Can you work these out from the model? Positions are in its coordinate system, mm. A direction names the side the tool comes from. Coordinates: 2 decimals unless noted, no trailing zeros. Write each loop counter-clockwise with the first axis right and the second up, starting at its lowest first coordinate (ties: lowest second). Pieces come first, ordered by that corner, then holes. Notation, with made-up numbers: M -13.75,26.25 L 16.25,26.25 A24 cw 16.25,40.25 Z; hole C 65.25,8.5 d6. An arc over 180 degrees is marked long. Answer as a JSON object with one key per item and string values. Group by question number.
from build123d import *

# Parameters (mm, degrees)
EXTRUDE_1_DEPTH     = 1.5
SKETCH_2_R          = 0.85
CUT_EXTRUDE_1_DEPTH = 11
SKETCH_4_R          = 0.85
CUT_EXTRUDE_2_DEPTH = 11.5
SKETCH_5_R          = 0.85
CUT_EXTRUDE_3_DEPTH = 11.5
SKETCH_9_R          = 1.55
SKETCH_9_R_2        = 0.85
CUT_EXTRUDE_5_DEPTH = 1
SKETCH_8_R          = 1.75
SKETCH_8_R_2        = 0.85
EXTRUDE_6_DEPTH     = 8.6
FILLET_2_R          = 1


with BuildPart() as part:
    # 草图1 → 凸台-拉伸1 (new body)
    with BuildSketch(Plane.XY):
        with BuildLine():
            Line((-26.273021583, 44.286870504), (15.826978417, 44.286870504))
            ThreePointArc((15.826978417, 44.286870504), (22.332360804, 41.592252891), (25.026978417, 35.086870504))
            Line((25.026978417, 35.086870504), (25.026978417, -7.013129496))
            ThreePointArc((25.026978417, -7.013129496), (22.332360804, -13.518511883), (15.826978417, -16.213129496))
            Line((15.826978417, -16.213129496), (-26.273021583, -16.213129496))
            ThreePointArc((-26.273021583, -16.213129496), (-32.77840397, -13.518511883), (-35.473021583, -7.013129496))
            Line((-35.473021583, -7.013129496), (-35.473021583, 35.086870504))
            ThreePointArc((-35.473021583, 35.086870504), (-32.77840397, 41.592252891), (-26.273021583, 44.286870504))
        make_face()
    extrude(amount=EXTRUDE_1_DEPTH)

    # 草图2 → 切除-拉伸1 (cut)
    with BuildSketch(Plane.XY.offset(1.5)):
        with Locations((-27.773021583, 36.586870504)):
            Circle(SKETCH_2_R)
    extrude(amount=-CUT_EXTRUDE_1_DEPTH, mode=Mode.SUBTRACT)

    # 草图4 → 切除-拉伸2 (cut)
    with BuildSketch(Plane.XY.offset(1.5)):
        with Locations((-27.773021583, -7.913129496)):
            Circle(SKETCH_4_R)
    extrude(amount=-CUT_EXTRUDE_2_DEPTH, mode=Mode.SUBTRACT)

    # 草图5 → 切除-拉伸3 (cut)
    with BuildSketch(Plane.XY.offset(1.5)):
        with Locations((17.326978417, -7.913129496)):
            Circle(SKETCH_5_R)
    extrude(amount=-CUT_EXTRUDE_3_DEPTH, mode=Mode.SUBTRACT)

    # 草图9 → 切除-拉伸5 (cut)
    # profile 1 of 3: a face of its own
    with BuildSketch(Plane.XY.offset(1.5)):
        with Locations((-27.773021583, 36.586870504)):
            Circle(SKETCH_9_R)
        with Locations((-27.773021583, 36.586870504)):
            Circle(SKETCH_9_R_2, mode=Mode.SUBTRACT)
    # profile 2 of 3: a face of its own
    with BuildSketch(Plane.XY.offset(1.5)):
        with Locations((-27.773021583, -7.913129496)):
            Circle(SKETCH_9_R)
        with Locations((-27.773021583, -7.913129496)):
            Circle(SKETCH_9_R_2, mode=Mode.SUBTRACT)
    # profile 3 of 3: a face of its own
    with BuildSketch(Plane.XY.offset(1.5)):
        with Locations((17.326978417, -7.913129496)):
            Circle(SKETCH_9_R)
        with Locations((17.326978417, -7.913129496)):
            Circle(SKETCH_9_R_2, mode=Mode.SUBTRACT)
    extrude(amount=-CUT_EXTRUDE_5_DEPTH, mode=Mode.SUBTRACT)

    # 草图8 → 凸台-拉伸6 (add)
    # profile 1 of 3: a face of its own
    with BuildSketch(Plane(origin=(0, 0, 0), x_dir=(-1, 0, 0), z_dir=(0, 0, -1))):
        with Locations(Location((27.773021583, 36.586870504, 0), (0, 0, 180))):
            Circle(SKETCH_8_R)
        with Locations(Location((27.773021583, 36.586870504, 0), (0, 0, 180))):
            Circle(SKETCH_8_R_2, mode=Mode.SUBTRACT)
    # profile 2 of 3: a face of its own
    with BuildSketch(Plane(origin=(0, 0, 0), x_dir=(-1, 0, 0), z_dir=(0, 0, -1))):
        with Locations(Location((27.773021583, -7.913129496, 0), (0, 0, 180))):
            Circle(SKETCH_8_R)
        with Locations(Location((27.773021583, -7.913129496, 0), (0, 0, 180))):
            Circle(SKETCH_8_R_2, mode=Mode.SUBTRACT)
    # profile 3 of 3: a face of its own
    with BuildSketch(Plane(origin=(0, 0, 0), x_dir=(-1, 0, 0), z_dir=(0, 0, -1))):
        with Locations(Location((-17.326978417, -7.913129496, 0), (0, 0, 180))):
            Circle(SKETCH_8_R)
        with Locations(Location((-17.326978417, -7.913129496, 0), (0, 0, 180))):
            Circle(SKETCH_8_R_2, mode=Mode.SUBTRACT)
    extrude(amount=EXTRUDE_6_DEPTH)

    # 圆角2
    fillet_2_edges = [part.edges().sort_by_distance(p)[0] for p in [
        (22.332360804, -13.518511883, 1.5),
        (25.026978417, 14.036870504, 1.5),
        (22.332360804, 41.592252891, 1.5),
        (-5.223021583, 44.286870504, 1.5),
        (-32.77840397, 41.592252891, 1.5),
        (-35.473021583, 14.036870504, 1.5),
        (-32.77840397, -13.518511883, 1.5),
        (-5.223021583, -16.213129496, 1.5),
    ]]
    fillet(fillet_2_edges, radius=FILLET_2_R)


solid = part.part
Q1. We'd pull the mould along X, two halves only. Please class faces 1 (the flat face through (-5, 14, 1.5)), 2 (the cylindrical face through (16.1, -8.86, 1.01)), 3 (the cylindrical face through (22.26, 41.663, 0.247)): pulls with the +X half, pulls with the -X half, needs draft (parallel to the pull), parting line crosses it, or undercut.
Q2. If we section it at B-B on y = 13.5: List the corners of the cut face in (x, z) for me.
Q3. If we section it at C-C on x = -15: List the corners of the cut face in (y, z) for me, and give its area (3 significant figures).
Q4. Will these pins go through, and if not, where does the flat tip stop? pin 1 (3 mm diameter, centred on x = 17.33, y = -7.91, fed in from +Z); pin 2 (2 mm diameter, centred on x = -27.77, y = 36.59, fed in from -Z); pin 3 (3 mm diameter, centred on x = -1.5, y = 20, fed in from -Z).
Q5. Please list where these lines run through material, in increasing order: L1, parallel to Y at x = 17.5, z = -4.75; L2, parallel to Z at x = 20, y = 34.5; L3, parallel to X at y = -7, z = -4.75.
Q6. If we section it at A-A on z = -4.75: List the corners of the cut face in (x, y) for me, and give its area (3 significant figures).
Q7. On a 3-axis mill with a long thin cutter (end or side, diameter ignored), from which of +Z, -Z, +X, -X, +Y, -Y can I reach the whole of each face in a straight line? I mean faces 4 (the cylindrical face through (-28.152, -6.205, -4.24)), 5 (the flat face through (-29, -8, -8.6)), 6 (the flat face through (-26.76, 36.61, 0.5)). Say none if no direction works.
Reply:
{
 "1": {"face 1": "needs draft", "face 2": "undercut", "face 3": "pulls with the +X half"},
 "2": {"outline": "M -35.47,0 L 25.03,0 L 25.03,0.5 A1 ccw 24.03,1.5 L -34.47,1.5 A1 ccw -35.47,0.5 Z"},
 "3": {"outline": "M -16.21,0 L 44.29,0 L 44.29,0.5 A1 ccw 43.29,1.5 L -15.21,1.5 A1 ccw -16.21,0.5 Z", "area": "90.3 mm^2"},
 "4": {"pin 1": "z = 0.5", "pin 2": "z = -8.6", "pin 3": "z = 0"},
 "5": {"L1": "-9.65 to -8.75, -7.08 to -6.17", "L2": "0 to 1.5", "L3": "-29.27 to -26.28, 15.83 to 18.82"},
 "6": {"outline": "C -27.77,-7.91 d3.5; C -27.77,36.59 d3.5; C 17.33,-7.91 d3.5; hole C -27.77,-7.91 d1.7; hole C -27.77,36.59 d1.7; hole C 17.33,-7.91 d1.7", "area": "22.1 mm^2"},
 "7": {"face 4": "-Z", "face 5": "-Z, +X, -X, +Y, -Y", "face 6": "+Z"}
}
